Study the drawing (mm; zero at the part's minimum x, y, z) and answer. A direction names the side the tool comes from. Coordinates: 2 decimals unless noted, no trailing zeros. Loops run counter-clockwise (first coordinate to the right, second up) from the corner with the lowest first, then second, coordinate; pieces in that order, holes last. Notation, with made-up numbers: (-21.5, 22) -> (33.5, 22) arc R14 cw to (33.5, 31) -> close; hole circle Ø3 at (54, 34). An arc over 180 degrees is marked (long way). Answer as CSV lines item,"result".
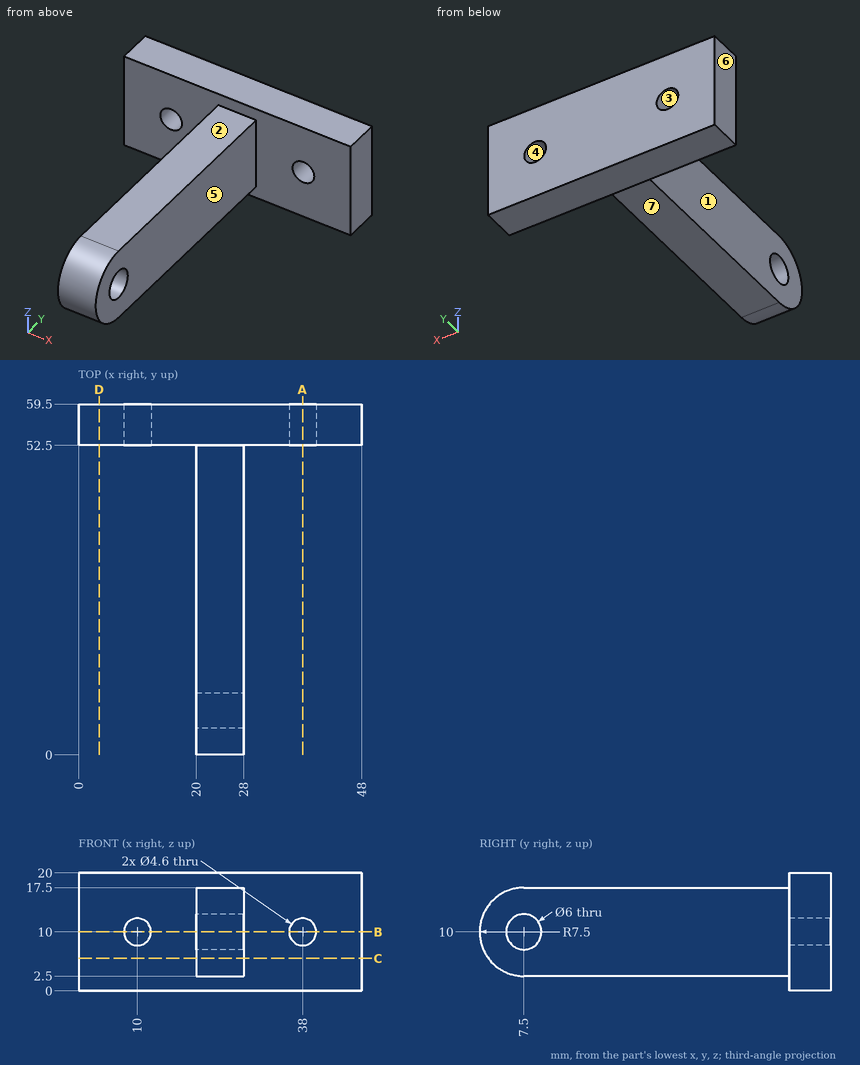
Q1. For the marked faces 1, 2 and 3, determine the directions among +Z, -Z, +X, -X, +Y, -Y from which every point of the face is accessible in a straight line to the end or side of a thin tool.
Results:
face 1,"+Z, -Z, -X, -Y"
face 2,"+Z, +X, -X, -Y"
face 3,"+Y, -Y"
Q2. A cutting plane is placed at D-D, the plane x = 3.5. Write down the section's boundary in (y, z).
Results:
outline,"(52.5, 0) -> (59.5, 0) -> (59.5, 20) -> (52.5, 20) -> close"
Q3. A cutting plane is placed at A-A, the plane x = 38. Write down the section's boundary in (y, z), and give its area (3 significant figures).
Results:
outline,"(52.5, 0) -> (59.5, 0) -> (59.5, 7.7) -> (52.5, 7.7) -> close; (52.5, 12.3) -> (59.5, 12.3) -> (59.5, 20) -> (52.5, 20) -> close"
area,"108 mm²"
Q4. Given pin 1 Ø4 at (y, z) = (37.5, 8) entering from +X; pin 2 Ø4 at (x, y) = (24.5, 25.5) entering from -Z; pin 3 Ø6 at (x, z) = (22.5, 17.5) entering from -Y, each flat-ended and moving along its own axis, determine where each tip first touches the part or whether it passes through.
Results:
pin 1,"stops at x = 28"
pin 2,"stops at z = 2.5"
pin 3,"stops at y = 1.5"
Q5. For a pull along X with two mould halves and no side action, classify the marked faces 4, 5, 6 and 7 as pulls with the +X half, pulls with the -X half, needs draft (parallel to the pull), parting line crosses it, or undercut.
Results:
face 4,"undercut"
face 5,"pulls with the +X half"
face 6,"pulls with the -X half"
face 7,"needs draft"
Q6. A cutting plane is placed at B-B, the plane z = 10. Write down the section's boundary in (x, y), and give its area (3 significant figures).
Results:
outline,"(0, 52.5) -> (7.7, 52.5) -> (7.7, 59.5) -> (0, 59.5) -> close; (12.3, 52.5) -> (20, 52.5) -> (20, 10.5) -> (28, 10.5) -> (28, 52.5) -> (35.7, 52.5) -> (35.7, 59.5) -> (12.3, 59.5) -> close; (20, 0) -> (28, 0) -> (28, 4.5) -> (20, 4.5) -> close; (40.3, 52.5) -> (48, 52.5) -> (48, 59.5) -> (40.3, 59.5) -> close"
area,"644 mm²"
Q7. A cutting plane is placed at C-C, the plane z = 5.5. Write down the section's boundary in (x, y).
Results:
outline,"(0, 52.5) -> (20, 52.5) -> (20, 1.5) -> (28, 1.5) -> (28, 52.5) -> (48, 52.5) -> (48, 59.5) -> (0, 59.5) -> close"
Q8. Find the intervals of material crossed by probe 1 along Z at (x, y) = (10, 55); probe 2 along Z at (x, y) = (26, 7.5); probe 3 along Y at (x, z) = (34, 2), in increasing order. Write a range as [from, to].
Results:
probe 1,"z = [0, 7.7], [12.3, 20]"
probe 2,"z = [2.5, 7], [13, 17.5]"
probe 3,"y = [52.5, 59.5]"
